from build123d import *

# Parameters (mm, degrees)
SKETCH_2_W             = 86.642852818
SKETCH_2_H             = 10
EXTRUDE_1_DEPTH        = 5.5
EXTRUDE_2_DEPTH        = 5
PATTERN_LINEAR_1_COUNT = 14
PATTERN_LINEAR_1_PITCH = 6.283185307
SKETCH_6_W             = 10
SKETCH_6_H             = 10
EXTRUDE_3_DEPTH        = 0.1
SKETCH_7_W             = 45
SKETCH_7_H             = 10
SKETCH_7_W_2           = 10
SKETCH_7_H_2           = 45
EXTRUDE_4_DEPTH        = 55


with BuildPart() as part:
    # 草图2 → 凸台-拉伸1 (new body)
    with BuildSketch(Plane(origin=(0, 0, 0), x_dir=(1, 0, 0), z_dir=(0, 1, 0))):
        Rectangle(SKETCH_2_W, SKETCH_2_H)
    extrude(amount=-EXTRUDE_1_DEPTH)

    # 草图3 → 凸台-拉伸2 (add, symmetric)
    with BuildSketch(Plane.XY):
        Polygon((-43.321426409, 0), (-41.683560355, 4.5), (-39.997848638, 4.5), (-38.359982584, 0), align=None)
    extrude_2 = extrude(amount=EXTRUDE_2_DEPTH, both=True)

    # 阵列(线性)1: 凸台-拉伸2 ×14
    with Locations(*[(i * PATTERN_LINEAR_1_PITCH, 0, 0) for i in range(1, PATTERN_LINEAR_1_COUNT)]):
        add(extrude_2)

    # 草图6 → 凸台-拉伸3 (add)
    with BuildSketch(Plane.ZY.offset(43.321426409)):
        with Locations((0, -0.5)):
            Rectangle(SKETCH_6_W, SKETCH_6_H)
    extrude(amount=EXTRUDE_3_DEPTH)

    # 草图7 → 凸台-拉伸4 (add)
    with BuildSketch(Plane.ZY.offset(43.421426409)):
        with Locations((27.5, -0.5)):
            Rectangle(SKETCH_7_W, SKETCH_7_H)
        with Locations((0, -0.5)):
            Rectangle(SKETCH_7_W_2, SKETCH_7_H)
        with Locations((0, 27)):
            Rectangle(SKETCH_7_W_2, SKETCH_7_H_2)
    extrude(amount=EXTRUDE_4_DEPTH)


solid = part.part
Geometry check sheet. Reference: the model listing, model coordinates, mm. A direction names the side the tool comes from. Coordinates: 2 decimals unless noted, no trailing zeros. Order: outer loops, then holes, each group sorted by start corner. A loop starts at its lowest first (then second) coordinate and runs counter-clockwise, first axis right, second up. Notation, with made-up numbers: (31.5, -25.5) - (86.5, -25.5) arc R21 ccw to (86.5, 7.5) - close; hole circle Ø7 at (-0.5, 22.5). An arc over 180 degrees is marked (long way). Answer in a Markdown table with one row per item. Add a question column.
1) Cross-section at B-B, the plane y = 29. Record the cut outline in (x, z), then the cut area to 3 significant figures.
2) Cross-section at A-A, the plane x = -58. Record the cut outline in (y, z), then the cut area to 3 significant figures.
3) Set-up check for faces 1 (the flat face through (-71, -1, 50)), 2 (the flat face through (-11.098, 2.218, 0.07)): record each of +Z, -Z, +X, -X, +Y, -Y from which the full face is reachable in a straight line by a thin tool's end or side.
4) Gauge pin test, flat ends, axial feed: P1, Ø0.8, axis at x = -22, z = -0.5, coming from the +Y side; P2, Ø1.1, axis at x = 12.5, z = -2, coming from the +Y side; P3, Ø5, axis at x = 12.5, y = 1, coming from the +Z side; P4, Ø3, axis at x = 6.5, y = 6.5, coming from the +Z side. Record the tip position at first contact, or that the pin passes through.
5) Release check for a two-part mould opening along X. For faces 3 (the flat face through (-43.421, 27, 0)), 4 (the flat face through (-71, 49.5, 0)), 5 (the flat face through (-23.664, 2.218, 0.07)) record: +X half, -X half, draft (parallel to the pull), parting line (faces both ways), or undercut.
6) Cross-section at C-C, the plane z = 41. Record the cut outline in (x, y).
7) Material ranges on line 1 along Z through (x, y) = (-59, 18.5); line 2 along X through (y, z) = (9, 1); line 3 along Y through (x, z) = (-53, 22.5), recorded low to high. Write a range as [from, to].
Check result:
| question | item | result |
|---|---|---|
| 1 | outline | (-98.42, -5) - (-43.42, -5) - (-43.42, 5) - (-98.42, 5) - close |
| 1 | area | 550 mm² |
| 2 | outline | (-5.5, -5) - (49.5, -5) - (49.5, 5) - (4.5, 5) - (4.5, 50) - (-5.5, 50) - close |
| 2 | area | 1,000 mm² |
| 3 | face 1 | +Z, +X, -X, +Y, -Y |
| 3 | face 2 | +Z, -Z, +Y |
| 4 | P1 | stops at y = 4.5 |
| 4 | P2 | stops at y = 0 |
| 4 | P3 | stops at z = 5 |
| 4 | P4 | passes through |
| 5 | face 3 | +X half |
| 5 | face 4 | draft |
| 5 | face 5 | undercut |
| 6 | outline | (-98.42, -5.5) - (-43.42, -5.5) - (-43.42, 4.5) - (-98.42, 4.5) - close |
| 7 | line 1 | z = [-5, 5] |
| 7 | line 2 | x = [-98.42, -43.42] |
| 7 | line 3 | y = [-5.5, 4.5] |
